Could you check a few things on this model? Use its own coordinates, in mm. Face numbers are marked on the shaded views. Coordinates: 2 decimals unless noted, no trailing zeros. Order: outer loops, then holes, each group sorted by start corner. A loop starts at its lowest first (then second) coordinate and runs counter-clockwise, first axis right, second up. Notation, with made-up numbers: (36, -6) -> (84, -6) arc R9 ccw to (84, 9) -> close; hole circle Ø8 at (-38.5, 32.25). An arc over 180 degrees is marked (long way). Use a Markdown table: item, result. Add a question column.
1) If we section it at A-A (y = 286): Write out the boundary of the cut face in (x, z).
2) Thinking about a two-plate mould opening in X: for the marked faces 1, 2 and 3, which applies, +X half, -X half, draft (parallel to the pull), parting line (faces both ways), or undercut?
3) If we section it at B-B (x = 559): Write out the boundary of the cut face in (y, z), plus the area to 3 significant figures.
4) Will this pin go through, and if not, where does the flat tip stop? pin 1 Ø2 at (x, y) = (289.5, 143) entering from +Z.
5) If I drill on L1, parallel to X at y = 310, z = 59; L2, parallel to Z at x = 1125, y = 209; L3, parallel to Z at x = 472, y = 374, over which ranges is the centre line in solid material (lowest first)? Write a range as [from, to].
6) If we section it at C-C (x = 1333.5): Write out the boundary of the cut face in (y, z).
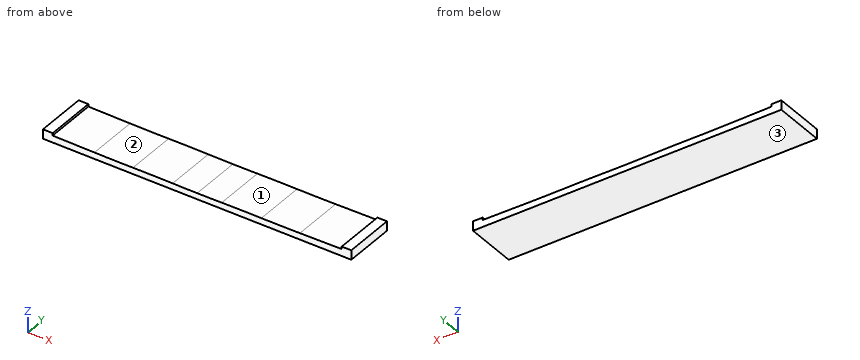
```python
from build123d import *

# Parameters (mm, degrees)
F1_DEPTH = 406.4


with BuildPart() as f1:
    # F0 (on Front) → F1 (new body)
    with BuildSketch(Plane.XZ):
        with BuildLine():
            Line((0, 55.52242), (0, 0))
            Line((0, 0), (2438.4, 0))
            Line((2438.4, 0), (2438.4, 55.52242))
            Line((2438.4, 55.52242), (2438.4, 74.573828))
            Line((2438.4, 74.573828), (2362.2, 73.647479))
            Line((2362.2, 73.647479), (2362.2, 54.596071))
            Line((2362.2, 54.596071), (2032, 50.581893))
            ThreePointArc((2032, 50.581893), (1879.601643, 49.491294), (1727.2, 49.924736))
            ThreePointArc((1727.2, 49.924736), (1570.312045, 50.347846), (1413.428048, 49.155868))
            ThreePointArc((1413.428048, 49.155868), (1316.315996, 48.227572), (1219.2, 47.918136))
            ThreePointArc((1219.2, 47.918136), (1122.084004, 48.227572), (1024.971952, 49.155868))
            ThreePointArc((1024.971952, 49.155868), (868.087955, 50.347846), (711.2, 49.924736))
            ThreePointArc((711.2, 49.924736), (558.798357, 49.491294), (406.4, 50.581893))
            Line((406.4, 50.581893), (76.2, 54.596071))
            Line((76.2, 54.596071), (76.2, 73.647479))
            Line((76.2, 73.647479), (0, 74.573828))
            Line((0, 74.573828), (0, 55.52242))
        make_face()
    extrude(amount=-F1_DEPTH)


solid = f1.part
```
Answer sheet:
| question | item | result |
|---|---|---|
| 1 | outline | (0, 0) -> (2438.4, 0) -> (2438.4, 74.57) -> (2362.2, 73.65) -> (2362.2, 54.6) -> (2032, 50.58) arc R15240.01 cw to (1727.2, 49.92) arc R15240 ccw to (1413.43, 49.16) arc R15239.99 cw to (1219.2, 47.92) arc R15239.99 cw to (1024.97, 49.16) arc R15240 ccw to (711.2, 49.92) arc R15240.01 cw to (406.4, 50.58) -> (76.2, 54.6) -> (76.2, 73.65) -> (0, 74.57) -> close |
| 2 | face 1 | undercut |
| 2 | face 2 | undercut |
| 2 | face 3 | draft |
| 3 | outline | (0, 0) -> (406.4, 0) -> (406.4, 49.49) -> (0, 49.49) -> close |
| 3 | area | 20,100 mm2 |
| 4 | pin 1 | z = 52.02 |
| 5 | L1 | [0, 76.2], [2362.2, 2438.4] |
| 5 | L2 | [0, 48.21] |
| 5 | L3 | [0, 49.93] |
| 6 | outline | (0, 0) -> (406.4, 0) -> (406.4, 48.35) -> (0, 48.35) -> close |
